Could you check a few things on this model? Use its own coordinates, in mm. Face numbers are marked on the shaded views. Round coordinates to 2 decimals unless told otherwise and drop trailing zeros. Order: outer loops, then holes, each group sorted by start corner. A loop starts at its lowest first (then second) coordinate and runs counter-clockwise, first axis right, second up. Notation, with made-up numbers: (-21.75, 42) -> (-16.75, 42) arc R10 ccw to (-16.75, 49) -> close; hole circle Ø4 at (3, -11.75). An arc over 180 degrees is marked (long way). One line per question, with ' | ' between items.
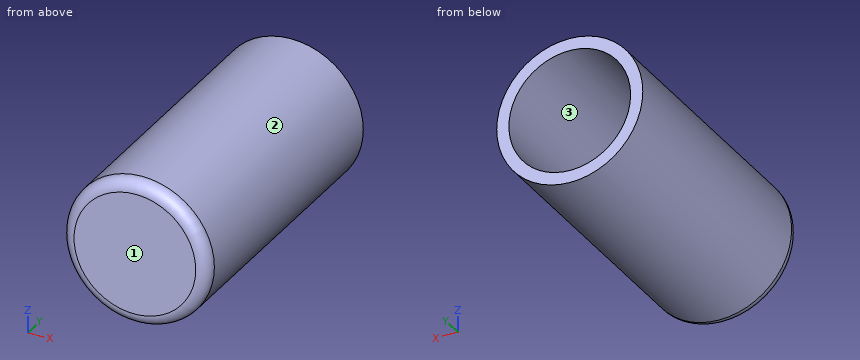
```python
from build123d import *

# Parameters (mm, degrees)
F0_R     = 30
F1_DEPTH = 120
F2_R     = 25
F3_DEPTH = 115
F4_R     = 5


with BuildPart() as f1:
    # F0 (on Front) → F1 (new body)
    with BuildSketch(Plane.XZ):
        Circle(F0_R)
    extrude(amount=F1_DEPTH)

    # F2 (on face) → F3 (cut)
    with BuildSketch(Plane(origin=(0, 0, 0), x_dir=(-1, 0, 0), z_dir=(0, 1, 0))):
        Circle(F2_R)
    extrude(amount=-F3_DEPTH, mode=Mode.SUBTRACT)

    # F4
    f4_edges = [f1.edges().sort_by_distance(p)[0] for p in [
        (-30, -120, 0),
    ]]
    fillet(f4_edges, radius=F4_R)


solid = f1.part
```
1. I want a section at A-A on x = 0. List the corners of the cut face in (y, z) for me, and give its area (3 significant figures).
From the geometry:
outline: (-120, -25) arc R5 ccw to (-115, -30) -> (0, -30) -> (0, -25) -> (-115, -25) -> (-115, 25) -> (0, 25) -> (0, 30) -> (-115, 30) arc R5 ccw to (-120, 25) -> close | area: 1,440 mm²
2. If we mould it in two halves opening along X, with no side actions, what happens to the marked faces 1, 2 and 3? For each: pulls with the +X half, pulls with the -X half, needs draft (parallel to the pull), parting line crosses it, or undercut.
From the geometry:
face 1: needs draft | face 2: parting line crosses it | face 3: undercut
3. I want a section at C-C on y = -81. List the corners of the cut face in (x, z) for me, and give its area (3 significant figures).
From the geometry:
outline: circle Ø60 at (0, 0); hole circle Ø50 at (0, 0) | area: 864 mm²
4. I need wall thicknesses on probe 1 along Z at (x, y) = (0, -74); probe 2 along Y at (x, z) = (-4.5, -4); probe 3 along Y at (x, z) = (-21, -14.5). Which ranges of each line are inside material? Lowest first, please.
From the geometry:
probe 1: z = -30 to -25, 25 to 30 | probe 2: y = -120 to -115 | probe 3: y = -119.97 to 0
5. I'm going to push flat-ended pins straight in: pin 1 (1 mm diameter, centred on x = -9.5, z = 6.5, fed in from +Y); pin 2 (1 mm diameter, centred on x = -17.5, z = 18.5, fed in from +Y); pin 3 (1 mm diameter, centred on y = -37.5, z = 5.5, fed in from -X); pin 4 (3 mm diameter, centred on y = -88, z = 11, fed in from +X). Where does each tip first touch, or does it pass through?
From the geometry:
pin 1: stops at y = -115 | pin 2: stops at y = 0 | pin 3: stops at x = -29.58 | pin 4: stops at x = 28.46
6. I want a section at B-B on z = 0. List the corners of the cut face in (x, y) for me, and give its area (3 significant figures).
From the geometry:
outline: (-30, -115) arc R5 ccw to (-25, -120) -> (25, -120) arc R5 ccw to (30, -115) -> (30, 0) -> (25, 0) -> (25, -115) -> (-25, -115) -> (-25, 0) -> (-30, 0) -> close | area: 1,440 mm²
